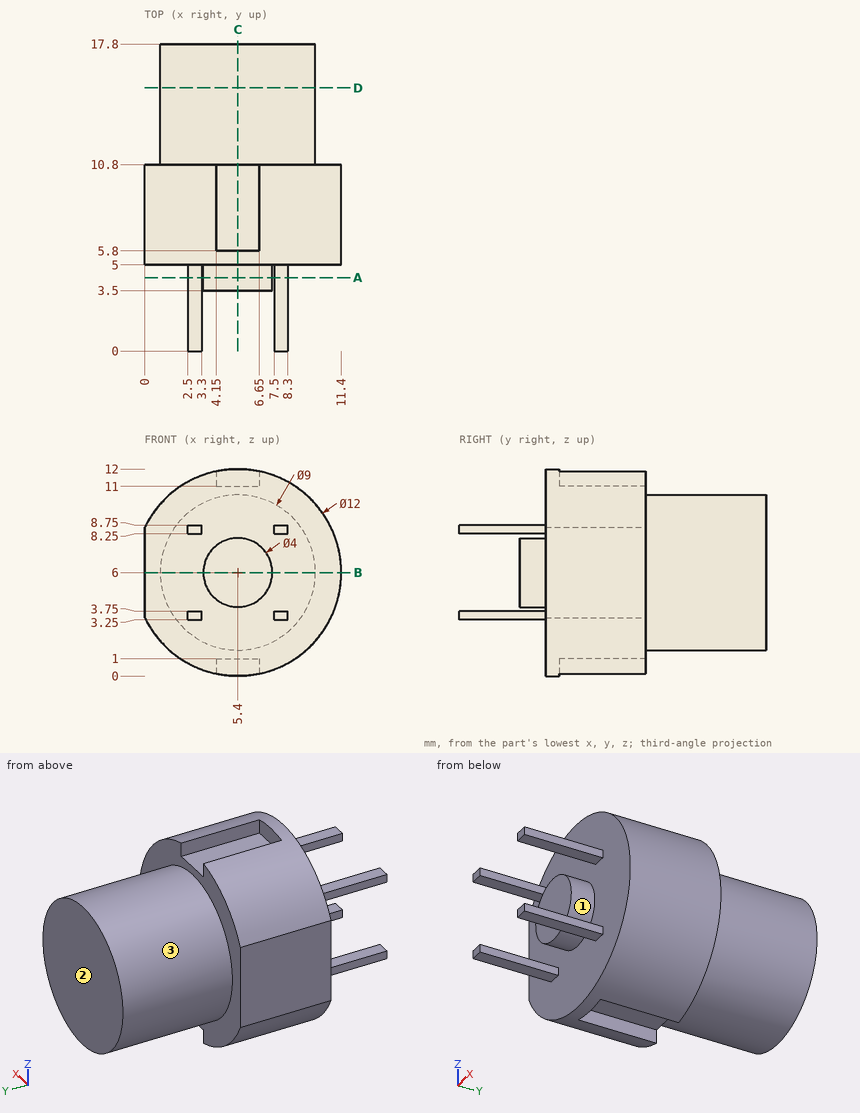
Here's the drawing with two shaded views (mm, measured from the low corner). I have some questions. A direction names the side the tool comes from. Round coordinates to 2 decimals unless told otherwise and drop trailing zeros. Order: outer loops, then holes, each group sorted by start corner. A loop starts at its lowest first (then second) coordinate and runs counter-clockwise, first axis right, second up. Notation, with made-up numbers: (79, -34) -> (87, -34) arc R16 cw to (87, -8) -> close; hole circle Ø9 at (-6, 64.5). An arc over 180 degrees is marked (long way). Return JSON: item names as keys, results as strings.
Q1. If we section it at D-D on y = 15.25: List the corners of the cut face in (x, z) for me, plus the area to 3 significant figures.
Filled sheet:
{"outline": "circle Ø9 at (5.4, 6)", "area": "63.6 mm^2"}
Q2. I need wall thicknesses on line 1 along Z through (x, y) = (8, 4); line 2 along Y through (x, z) = (2.25, 8.75); line 3 along Y through (x, z) = (8.5, 10.75). Which ranges of each line are inside material? Lowest first, please. Write a range as from..to.
Filled sheet:
{"line 1": "z = 3.25..3.75, 8.25..8.75", "line 2": "y = 5..17.8", "line 3": "y = 5..10.8"}
Q3. If we section it at B-B on z = 6: List the corners of the cut face in (x, y) for me, plus the area to 3 significant figures.
Filled sheet:
{"outline": "(0, 5) -> (3.4, 5) -> (3.4, 3.5) -> (7.4, 3.5) -> (7.4, 5) -> (11.4, 5) -> (11.4, 10.8) -> (9.9, 10.8) -> (9.9, 17.8) -> (0.9, 17.8) -> (0.9, 10.8) -> (0, 10.8) -> close", "area": "135 mm^2"}
Q4. If we section it at A-A on y = 4.25: List the corners of the cut face in (x, z) for me, plus the area to 3 significant figures.
Filled sheet:
{"outline": "(2.5, 3.25) -> (3.3, 3.25) -> (3.3, 3.75) -> (2.5, 3.75) -> close; (2.5, 8.25) -> (3.3, 8.25) -> (3.3, 8.75) -> (2.5, 8.75) -> close; circle Ø4 at (5.4, 6); (7.5, 3.25) -> (8.3, 3.25) -> (8.3, 3.75) -> (7.5, 3.75) -> close; (7.5, 8.25) -> (8.3, 8.25) -> (8.3, 8.75) -> (7.5, 8.75) -> close", "area": "14.2 mm^2"}
Q5. Which directions (+Z, -Z, +X, -X, +Y, -Y) give clear straight access to the entire face, cutting with the end or side of a thin tool? Please do the marked faces 1, 2 and 3.
Filled sheet:
{"face 1": "-Y", "face 2": "+Z, -Z, +X, -X, +Y", "face 3": "+Y"}
Q6. If we section it at C-C on x = 5.4: List the corners of the cut face in (y, z) for me, plus the area to 3 significant figures.
Filled sheet:
{"outline": "(3.5, 4) -> (5, 4) -> (5, 0) -> (5.8, 0) -> (5.8, 1) -> (10.8, 1) -> (10.8, 1.5) -> (17.8, 1.5) -> (17.8, 10.5) -> (10.8, 10.5) -> (10.8, 11) -> (5.8, 11) -> (5.8, 12) -> (5, 12) -> (5, 8) -> (3.5, 8) -> close", "area": "129 mm^2"}
Q7. For pin 1 Ø3 at (x, z) = (5, 6) entering from -Y; pin 2 Ø0.5 at (x, z) = (5.5, 11.5) entering from +Y; pin 3 Ø5 at (x, y) = (9.5, 4.5) entering from +Z, each with a flat end and sliding along its axis, tell me the tip position at first contact or that it passes through.
Filled sheet:
{"pin 1": "stops at y = 3.5", "pin 2": "stops at y = 5.8", "pin 3": "stops at z = 11.77"}
